Can you work these out from the model? Positions are in its coordinate system, mm. A direction names the side the tool comes from. Coordinates: 2 decimals unless noted, no trailing zeros. Write each loop counter-clockwise with the first axis right and the second up, starting at its lowest first coordinate (ties: lowest second). Pieces come first, ordered by that corner, then holes. Notation, with made-up numbers: M 41,27.25 L 85,27.25 A31 ccw 85,60.25 Z; hole C 67.25,-25 d1. An arc over 180 degrees is marked long. Use one line per item in the form item = value. Start each with the question number.
```python
from build123d import *

# Parameters (mm, degrees)
BOSS_EXTRUDE1_DEPTH = 0.6
SKETCH2_W           = 4
SKETCH2_H           = 2
BOSS_EXTRUDE2_DEPTH = 0.6
FILLET1_R           = 0.3
SKETCH5_W           = 0.5
SKETCH5_H           = 0.75
BOSS_EXTRUDE3_DEPTH = 0.25
FILLET2_R           = 0.25


with BuildPart() as part:
    # Sketch1 → Boss-Extrude1 (new body)
    with BuildSketch(Plane(origin=(0, 0, 0), x_dir=(1, 0, 0), z_dir=(0, 1, 0))):
        Polygon((0, 0), (0, 5), (1, 5), (1, 9.5), (0, 9.5), (0, 6), (-2, 6), (-2, 6.5), (-6, 6.5), (-6, 5), (-1, 5), (-1, 0), align=None)
    extrude(amount=BOSS_EXTRUDE1_DEPTH)



with BuildPart() as body_2:
    # Sketch2 → Boss-Extrude2 (new body)
    with BuildSketch(Plane(origin=(0, 0.6, 0), x_dir=(1, 0, 0), z_dir=(0, 1, 0))):
        with Locations((-4, 8.5)):
            Rectangle(SKETCH2_W, SKETCH2_H)
    extrude(amount=BOSS_EXTRUDE2_DEPTH)


with BuildPart() as part_1:
    add(part.part)

    add(body_2.part)  # Loft1 merges body 2
    # Sketch3 → Loft1 section 0
    with BuildSketch(Plane.XY.offset(-7.5)):
        with BuildLine():
            Line((-3, 1.2), (-5, 1.2))
            Line((-5, 1.2), (-5, 0.6))
            Line((-5, 0.6), (-3, 0.6))
            Line((-3, 0.6), (-3, 1.2))
        make_face()
    # Sketch4 → Loft1 section 1
    with BuildSketch(Plane(origin=(0, 0, -6.5), x_dir=(-1, 0, 0), z_dir=(0, 0, -1))):
        with BuildLine():
            Line((3, 0.6), (5, 0.6))
            Line((5, 0.6), (5, 0))
            Line((5, 0), (3, 0))
            Line((3, 0), (3, 0.6))
        make_face()
    loft()

    # Fillet1
    fillet1_edges = [part_1.edges().sort_by_distance(p)[0] for p in [
        (-1, 0.3, 0),
        (0, 0.3, 0),
    ]]
    fillet(fillet1_edges, radius=FILLET1_R)

    # Sketch5 → Boss-Extrude3 (add)
    with BuildSketch(Plane(origin=(0, 1.2, 0), x_dir=(1, 0, 0), z_dir=(0, 1, 0))):
        with Locations((-4, 9.125)):
            Rectangle(SKETCH5_W, SKETCH5_H)
    extrude(amount=BOSS_EXTRUDE3_DEPTH)

    # Fillet2
    fillet2_edges = [part_1.edges().sort_by_distance(p)[0] for p in [
        (-3.75, 1.45, -9.125),
        (-4.25, 1.45, -9.125),
    ]]
    fillet(fillet2_edges, radius=FILLET2_R - 0.0001)  # a hair under: the kernel refuses the full size


solid = part_1.part
```
1) Suppose I cut it at D-D on z = -4. Please give me the cut outline in (x, y), and give its area (3 significant figures).
2) Suppose I cut it at B-B on z = -6.25. Please give me the cut outline in (x, y), and give its area (3 significant figures).
3) Will these pins go through, and if not, where does the flat tip stop? pin 1 Ø3 at (x, z) = (0, -1.5) entering from +Y; pin 2 Ø0.5 at (x, y) = (0.5, 0.5) entering from +Z; pin 3 Ø0.7 at (y, z) = (1, -9) entering from +X.
4) Which directions (+Z, -Z, +X, -X, +Y, -Y) give clear straight access to the entire face, cutting with the end or side of a thin tool? Please do faces 1 (the face through (-1.2, 0.6, -5.5)), 2 (the face through (-4, 0.3, -7)), 3 (the face through (-4, 1, -9.5)).
5) Suppose I cut it at C-C on x = -1.25. Please give me the cut outline in (y, z).
6) Suppose I cut it at A-A on x = -2.75. Please give me the cut outline in (y, z), and give its area (3 significant figures).
7) Please list where these lines run through material, in increasing order: line 1 (Y direction, x = -5.5, z = -8.25); line 2 (Z direction, x = -5.5, y = 0.45); line 3 (X direction, y = 0.15, z = -7.25).
Computed values:
q1.outline = M -1,0 L 0,0 L 0,0.6 L -1,0.6 Z
q1.area = 0.600 mm²
q2.outline = M -6,0 L -2,0 L -2,0.6 L -6,0.6 Z; M 0,0 L 1,0 L 1,0.6 L 0,0.6 Z
q2.area = 3.00 mm²
q3.pin_1 = 0.6
q3.pin_2 = -5
q3.pin_3 = -2
q4.face_1 = +Z, +X, +Y
q4.face_2 = -Z, -X, -Y
q4.face_3 = -Z, +X, -X, +Y, -Y
q5.outline = M 0,-6 L 0.6,-6 L 0.6,-5 L 0,-5 Z
q6.outline = M 0,-6.5 L 0.6,-6.5 L 0.6,-5 L 0,-5 Z; M 0.6,-9.5 L 1.2,-9.5 L 1.2,-7.5 L 0.6,-7.5 Z
q6.area = 2.10 mm²
q7.line_1 = 0.6 to 1.2
q7.line_2 = -6.5 to -5
q7.line_3 = 0 to 1
